Can you work these out from the model? Positions are in its coordinate system, mm. Coordinates: 2 decimals unless noted, no trailing zeros. Loops run counter-clockwise (first coordinate to the right, second up) from the corner with the lowest first, then second, coordinate; pieces in that order, holes last. Notation, with made-up numbers: (38, 1.5) -> (70, 1.5) arc R23 ccw to (70, 20.5) -> close; hole circle Ø4 at (37.5, -38.5). An arc over 180 degrees is marked (long way). Put each result on its own line as item: value. Start each with the question number.
Item 1: If we section it at C-C on x = 599: Please give me the cut outline in (y, z).
Item 2: Will these pins go through, and if not, where does the flat tip stop? P1, Ø1.5, axis at y = 77, z = 1, coming from the -X side; P2, Ø5, axis at y = -29, z = 3, coming from the -X side.
Item 3: If we section it at A-A on z = -3.25: Please give me the cut outline in (x, y), plus the area to 3 significant figures.
Item 4: Please list where these lines run through material, in increasing order: L1, parallel to Y at x = 653, z = -4; L2, parallel to X at y = 2.5, z = -6.5; L3, parallel to Y at x = -578, z = -2.5. Write a range as from..to.
Item 5: If we section it at B-B on y = 0.5: Please give me the cut outline in (x, z).
```python
from build123d import *

# Parameters (mm, degrees)
F1_DEPTH = 8


# Not quite as in the source:
# - ends of sketch curves that miss each other by under 0.0002 mm in the source are joined


with BuildPart() as f1:
    # F0 (on Top) → F1 (new body, symmetric)
    with BuildSketch(Plane.XY):
        with BuildLine():
            Line((-475, 65), (-475, -65))
            Line((-475, -65), (-810, -65))
            Line((-810, -65), (-810, -68.972132))
            ThreePointArc((-810, -68.972132), (-798.6528240235, -100.6889917911), (-769.7616321997, -118.0099800033))
            Line((-769.7616321997, -118.0099800033), (-397.046108, -192.203936))
            ThreePointArc((-397.046108, -192.203936), (-383.3390652577, -195.9623660974), (-370.3033040103, -201.6260880198))
            Line((-370.3033040103, -201.6260880198), (-221.58307, -279.239461))
            ThreePointArc((-221.58307, -279.239461), (-206.5717643435, -284.2486537093), (-190.746885103, -284.3157393396))
            Line((-190.746885103, -284.3157393396), (342.343109, -201.193898))
            ThreePointArc((342.343109, -201.193898), (350.023164587, -200.2989211876), (357.749411, -200))
            Line((357.749411, -200), (810, -200))
            Line((810, -200), (810, 200))
            Line((810, 200), (357.749411, 200))
            ThreePointArc((357.749411, 200), (350.023164587, 200.2989211876), (342.343108949, 201.1938976727))
            Line((342.343108949, 201.1938976727), (-190.746885, 284.31574))
            ThreePointArc((-190.746885, 284.31574), (-206.5717643435, 284.2486537093), (-221.5830694776, 279.2394599991))
            Line((-221.5830694776, 279.2394599991), (-370.303304, 201.626088))
            ThreePointArc((-370.303304, 201.626088), (-383.3390652577, 195.9623660974), (-397.0461080216, 192.2039361086))
            Line((-397.0461080216, 192.2039361086), (-769.761632, 118.009979))
            ThreePointArc((-769.761632, 118.009979), (-798.6528240235, 100.6889917911), (-810, 68.972132))
            Line((-810, 68.972132), (-810, 65))
            Line((-810, 65), (-475, 65))
        make_face()
    extrude(amount=F1_DEPTH, both=True)


solid = f1.part
```
Solutions:
1. outline: (-200, -8) -> (200, -8) -> (200, 8) -> (-200, 8) -> close
2. P1: x = -809.47
2. P2: x = -475
3. outline: (-810, -68.97) arc R50 ccw to (-769.76, -118.01) -> (-397.05, -192.2) arc R100 cw to (-370.3, -201.63) -> (-221.58, -279.24) arc R50 ccw to (-190.75, -284.32) -> (342.34, -201.19) arc R100 cw to (357.75, -200) -> (810, -200) -> (810, 200) -> (357.75, 200) arc R100 cw to (342.34, 201.19) -> (-190.75, 284.32) arc R50 ccw to (-221.58, 279.24) -> (-370.3, 201.63) arc R100 cw to (-397.05, 192.2) -> (-769.76, 118.01) arc R50 ccw to (-810, 68.97) -> (-810, 65) -> (-475, 65) -> (-475, -65) -> (-810, -65) -> close
3. area: 626,000 mm^2
4. L1: -200..200
4. L2: -475..810
4. L3: -156.18..-65, 65..156.18
5. outline: (-475, -8) -> (810, -8) -> (810, 8) -> (-475, 8) -> close
